from build123d import *

# Parameters (mm, degrees)
F1_DEPTH = 50.8
F2_R     = 9.525
F4_DEPTH = 38.101
F3_R     = 4.826
F5_DEPTH = 38.101
F3_W     = 15.875
F3_H     = 15.875
F8_DEPTH = 10.16
F9_R     = 1.6002


with BuildPart() as f1:
    # F0 (on Front) → F1 (new body)
    with BuildSketch(Plane.XZ):
        Polygon((0, 33.3248), (0, 0), (33.3248, 0), (33.3248, -4.7752), (38.1, -4.7752), (38.1, 33.3248), align=None)
    extrude(amount=F1_DEPTH)

    # F2 (on face) → F4 (cut, through all)
    with BuildSketch(Plane.YZ.offset(38.1)):
        with Locations((-25.4, 19.05)):
            Circle(F2_R)
    extrude(amount=-F4_DEPTH, mode=Mode.SUBTRACT)

    # F3 (on face) → F5 (cut, through all)
    with BuildSketch(Plane.XY.offset(33.3248)):
        with Locations((17.4498, -9.525)):
            Circle(F3_R)
        with Locations((17.4498, -41.275)):
            Circle(F3_R)
    extrude(amount=-F5_DEPTH, mode=Mode.SUBTRACT)

    # F3 (on face) → F8 (cut)
    with BuildSketch(Plane.XY.offset(33.3248)):
        with Locations((17.4498, -11.1125)):
            Rectangle(F3_W, F3_H)
        with Locations((17.4498, -9.525)):
            Circle(F3_R, mode=Mode.SUBTRACT)
        with Locations((17.4498, -39.6875)):
            Rectangle(F3_W, F3_H)
        with Locations((17.4498, -41.275)):
            Circle(F3_R, mode=Mode.SUBTRACT)
    extrude(amount=-F8_DEPTH, mode=Mode.SUBTRACT)

    # F9
    f9_edges = [f1.edges().sort_by_distance(p)[0] for p in [
        (9.5123, -47.625, 28.2448),
        (9.5123, -31.75, 29.737158),
        (9.5123, -3.175, 28.2448),
        (9.5123, -19.05, 29.737158),
        (25.3873, -19.05, 29.737158),
        (25.3873, -47.625, 28.2448),
        (25.3873, -31.75, 29.737158),
        (25.3873, -3.175, 28.2448),
    ]]
    fillet(f9_edges, radius=F9_R)


solid = f1.part
The listing builds one solid part. Answer for the finished solid, in the listing's coordinates (mm). A direction names the side the tool comes from. Round coordinates to 2 decimals unless told otherwise and drop trailing zeros. Loops run counter-clockwise (first coordinate to the right, second up) from the corner with the lowest first, then second, coordinate; pieces in that order, holes last. Notation, with made-up numbers: M 66,-0.5 L 105,-0.5 A13 ccw 105,23.5 Z; hole C 34,11 d7. An arc over 180 degrees is marked long. Return JSON: item names as keys, results as strings.
Q1. The mould has two halves that part along X. Classify faces 3 (the face through (16.82, -4.74, 11.74)), 4 (the face through (33.325, -25, -2)), 5 (the face through (16, -25, 0)), 6 (the face through (17, -36, 23.165)): released by +X, released by -X, zero draft, split by the parting line, or undercut.
Results list:
{"face 3": "undercut", "face 4": "released by -X", "face 5": "zero draft", "face 6": "undercut"}
Q2. Each of these flat-tipped pins is pushed along its axis until it touches: pin 1 Ø2 at (x, z) = (18, 29) entering from +Y; pin 2 Ø4 at (x, y) = (19, -8) entering from +Z; pin 3 Ø11 at (x, y) = (17.45, -9.52) entering from +Z; pin 4 Ø1.4 at (y, z) = (-31, -2) entering from -X. Where does it stop, or does it pass through?
Results list:
{"pin 1": "stops at y = 0", "pin 2": "passes through", "pin 3": "stops at z = 23.16", "pin 4": "stops at x = 33.32"}
Q3. Find section D-D, the plane z = 19.05. Determine the outline of the cut face in (x, y) (3 decimals).
Results list:
{"outline": "M 0,-50.8 L 38.1,-50.8 L 38.1,-34.925 L 0,-34.925 Z; M 0,-15.875 L 38.1,-15.875 L 38.1,0 L 0,0 Z; hole C 17.45,-41.275 d9.652; hole C 17.45,-9.525 d9.652"}
Q4. Find section C-C, the plane y = -25.4. Determine the outline of the cut face in (x, z) (3 decimals).
Results list:
{"outline": "M 0,0 L 33.325,0 L 33.325,-4.775 L 38.1,-4.775 L 38.1,9.525 L 0,9.525 Z; M 0,28.575 L 38.1,28.575 L 38.1,33.325 L 0,33.325 Z"}
Q5. Which of the six approach directions +Z, -Z, +X, -X, +Y, -Y give full straight-line access (tool end or side, diameter ignored) to faces 1 (the face through (36, -25, -4.775)), 2 (the face through (24.931, -47.144, 28.174))?
Results list:
{"face 1": "-Z, +X, -X, +Y, -Y", "face 2": "+Z"}
Q6. Find section B-B, the plane x = 5.5. Determine the outline of the cut face in (y, z) (3 decimals).
Results list:
{"outline": "M -50.8,0 L 0,0 L 0,33.325 L -50.8,33.325 Z; hole C -25.4,19.05 d19.05"}
Q7. Find section A-A, the plane z = 30. State how many separate pieces and enclosed holes the cut face has, plus the area to 3 significant figures.
Results list:
{"separate pieces": "1", "enclosed holes": "2", "area": "1,440 mm2"}
Q8. Find the intervals of material crossed by line 1 along Z through (x, y) = (25, -25); line 2 along X through (y, z) = (-35.5, 24); line 3 along Y through (x, z) = (18, 19), in increasing order. Write a range as from..to.
Results list:
{"line 1": "z = 0..9.53, 28.57..33.32", "line 2": "x = 0..9.51, 25.39..38.1", "line 3": "y = -50.8..-46.07, -36.48..-34.92, -15.88..-14.32, -4.73..0"}
